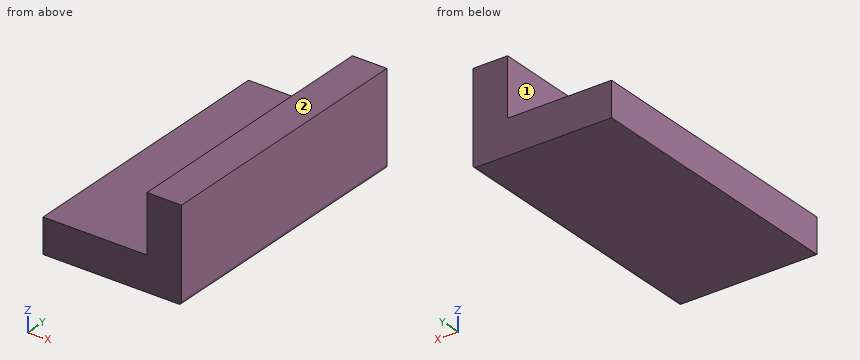
```python
from build123d import *

# Parameters (mm, degrees)
F0_W     = 57.15
F0_H     = 19.05
F1_DEPTH = 152.4


with BuildPart() as f1:
    # F0 (on Front) → F1 (new body)
    with BuildSketch(Plane.XZ):
        with Locations((-9.525, -15.875)):
            Rectangle(F0_W, F0_H)
        with BuildLine():
            ThreePointArc((36.5125, -25.4), (37.635032, -24.935032), (38.1, -23.8125))
            Line((38.1, -23.8125), (38.1, 25.4))
            Line((38.1, 25.4), (19.05, 25.4))
            Line((19.05, 25.4), (19.05, -6.35))
            Line((19.05, -6.35), (19.05, -25.4))
            Line((19.05, -25.4), (36.5125, -25.4))
        make_face()
    extrude(amount=F1_DEPTH)


solid = f1.part
```
Here's how the part is built. I have some questions about the finished solid (model axes, mm). Face numbers are marked on the shaded views. A direction names the side the tool comes from. Coordinates: 2 decimals unless noted, no trailing zeros. Order: outer loops, then holes, each group sorted by start corner. A loop starts at its lowest first (then second) coordinate and runs counter-clockwise, first axis right, second up. Notation, with made-up numbers: (-26, 77.25) -> (-13, 77.25) arc R21 ccw to (-13, 110.25) -> close; hole circle Ø6 at (29, 76.5). An arc over 180 degrees is marked (long way). Return JSON: item names as keys, results as strings.
1) If I drill on probe 1 along Z at (x, y) = (18, -103); probe 2 along X at (y, z) = (-52, 19.5), over which ranges is the centre line in solid material (lowest first)?
Conclusion:
{"probe 1": "z = -25.4 to -6.35", "probe 2": "x = 19.05 to 38.1"}
2) If we section it at B-B on z = 4: List the corners of the cut face in (x, y) for me, plus the area to 3 significant figures.
Conclusion:
{"outline": "(19.05, -152.4) -> (38.1, -152.4) -> (38.1, 0) -> (19.05, 0) -> close", "area": "2,900 mm²"}
3) I'm going to push flat-ended pins straight in: P1, Ø3, axis at x = 12, y = -59.5, coming from the +Z side; P2, Ø16, axis at y = -100.5, z = 12, coming from the -X side. Where does each tip first touch, or does it pass through?
Conclusion:
{"P1": "stops at z = -6.35", "P2": "stops at x = 19.05"}
4) On a 3-axis mill with a long thin cutter (end or side, diameter ignored), from which of +Z, -Z, +X, -X, +Y, -Y can I reach the whole of each face in a straight line? I mean the marked faces 1 and 2. Say none if no direction works.
Conclusion:
{"face 1": "+Z, -X, +Y, -Y", "face 2": "+Z, +X, -X, +Y, -Y"}
5) If we section it at C-C on x = -17: List the corners of the cut face in (y, z) for me.
Conclusion:
{"outline": "(-152.4, -25.4) -> (0, -25.4) -> (0, -6.35) -> (-152.4, -6.35) -> close"}
